from build123d import *

# Parameters (mm, degrees)
F0_W     = 20
F0_H     = 70
F1_DEPTH = 20
F2_W     = 4
F2_H     = 70
F3_DEPTH = 15
F4_R     = 2


with BuildPart() as f1:
    # F0 (on Top) → F1 (new body)
    with BuildSketch(Plane.XY):
        Rectangle(F0_W, F0_H)
    extrude(amount=F1_DEPTH)

    # F2 (on face) → F3 (cut)
    with BuildSketch(Plane.XY.offset(20)):
        with Locations((-4, 0)):
            Rectangle(F2_W, F2_H)
    extrude(amount=-F3_DEPTH, mode=Mode.SUBTRACT)

    # F4
    f4_edges = [f1.edges().sort_by_distance(p)[0] for p in [
        (10, 0, 20),
        (-10, 0, 20),
        (4, -35, 20),
        (-8, -35, 20),
        (4, 35, 20),
        (-8, 35, 20),
        (10, -35, 10),
        (-10, -35, 10),
        (10, 35, 10),
        (-10, 35, 10),
    ]]
    fillet(f4_edges, radius=F4_R)


solid = f1.part
Read the model definition and answer for the solid it produces. Units are mm, in the model's axes. A direction names the side the tool comes from. Give positions to 0.01 mm unless a question says otherwise; leave off trailing zeros. Loops run counter-clockwise (first coordinate to the right, second up) from the corner with the lowest first, then second, coordinate; pieces in that order, holes last. Notation, with made-up numbers: (37.25, 20.5) -> (50.25, 20.5) arc R21 ccw to (50.25, 59.5) -> close; hole circle Ø9 at (27, 27.5). An arc over 180 degrees is marked (long way). Use a Markdown table: item, result.
Q1. Section B-B, the plane y = -21.5 is taken. Determine the outline of the cut face in (x, z).
Solved:
| item | result |
|---|---|
| outline | (-10, 0) -> (10, 0) -> (10, 18) arc R2 ccw to (8, 20) -> (-2, 20) -> (-2, 5) -> (-6, 5) -> (-6, 20) -> (-8, 20) arc R2 ccw to (-10, 18) -> close |
Q2. A tool of negligible diameter and unlimited length cuts with its end or side. For faces 4 (the face through (-2, 0, 13)), 5 (the face through (-9.43, -34.4, 9.13)), from which of +Z, -Z, +X, -X, +Y, -Y can it reach the whole face along a straight path? Write none if from no direction.
Solved:
| item | result |
|---|---|
| face 4 | +Z, +Y, -Y |
| face 5 | +Z, -Z, -X, -Y |
Q3. This flat-tipped pin is pushed along its axis until it touches: pin 1 (2 mm diameter, centred on x = -4, y = -12, fed in from +Z). Where does it stop, or does it pass through?
Solved:
| item | result |
|---|---|
| pin 1 | stops at z = 5 |
Q4. Section A-A, the plane z = 6 is taken. Determine the outline of the cut face in (x, y), then the cut area to 3 significant figures.
Solved:
| item | result |
|---|---|
| outline | (-10, -33) arc R2 ccw to (-8, -35) -> (-6, -35) -> (-6, 35) -> (-8, 35) arc R2 ccw to (-10, 33) -> close; (-2, -35) -> (8, -35) arc R2 ccw to (10, -33) -> (10, 33) arc R2 ccw to (8, 35) -> (-2, 35) -> close |
| area | 1,120 mm^2 |
Q5. Section C-C, the plane x = -3.75 is taken. Determine the outline of the cut face in (y, z), then the cut area to 3 significant figures.
Solved:
| item | result |
|---|---|
| outline | (-35, 0) -> (35, 0) -> (35, 5) -> (-35, 5) -> close |
| area | 350 mm^2 |
Q6. Find the intervals of material crossed by line 1 along X through (y, z) = (-30, 5.5); line 2 along Z through (x, y) = (8.25, 5); line 3 along Z through (x, y) = (-5.5, -24), in increasing order.
Solved:
| item | result |
|---|---|
| line 1 | x = -10 to -6, -2 to 10 |
| line 2 | z = 0 to 19.98 |
| line 3 | z = 0 to 5 |
Q7. Determine the mould class of faces 1 (the face through (9.4, 34.43, 9.13)), 2 (the face through (-6, 0, 13)), 3 (the face through (0, 0, 0)) for opening direction X: pulls with the +X half, pulls with the -X half, needs draft (parallel to the pull), parting line crosses it, or undercut.
Solved:
| item | result |
|---|---|
| face 1 | pulls with the +X half |
| face 2 | undercut |
| face 3 | needs draft |
